Job drawing, mm, ordinate dimensions from the low corner. One solid piece. A direction names the side the tool comes from. Round coordinates to 2 decimals unless told otherwise and drop trailing zeros. Loops run counter-clockwise (first coordinate to the right, second up) from the corner with the lowest first, then second, coordinate; pieces in that order, holes last. Notation, with made-up numbers: M 13.25,77.25 L 33.25,77.25 A21 ccw 33.25,92.25 Z; hole C -24.75,77 d7. An arc over 180 degrees is marked long. Use a Markdown table: item, result. Add a question column.
(1) Flat gauge pins, fed straight in: P1, Ø1.8, axis at x = 20, z = 12.5, coming from the +Y side; P2, Ø7, axis at x = 20, z = 11, coming from the -Y side; P3, Ø4.5, axis at x = 7, y = 5.5, coming from the +Z side; P4, Ø2, axis at x = 22.5, y = 9, coming from the +Z side. Where does each tip first touch, or does it go through?
(2) Band-saw the part on C-C, the plane y = 3.5. Write the cut outline in (x, z).
(3) Which spindle directions (+Z, -Z, +X, -X, +Y, -Y) get a long thin tool onto all of the face, cutting with end or side? Do the marked faces 4, 5, 6 and 7. Say none if no direction does.
(4) Two-plate mould, pull along Z, no slides. Class the marked faces 1, 2 and 3: released by +Z, released by -Z, zero draft, split by the parting line, or undercut.
(5) Band-saw the part on B-B, the plane z = 11. Give the number of separate pieces and of enclosed holes in the cut face, and give its area (3 significant figures).
(6) Band-saw the part on A-A, the plane x = 5. Write the cut outline in (y, z).
(7) Wall check: L1, parallel to X at y = 9.3, z = 11; L2, parallel to X at y = 2, z = 11; L3, parallel to X at y = 4.75, z = 8.25. Give the ranges that are in metal, low to high.
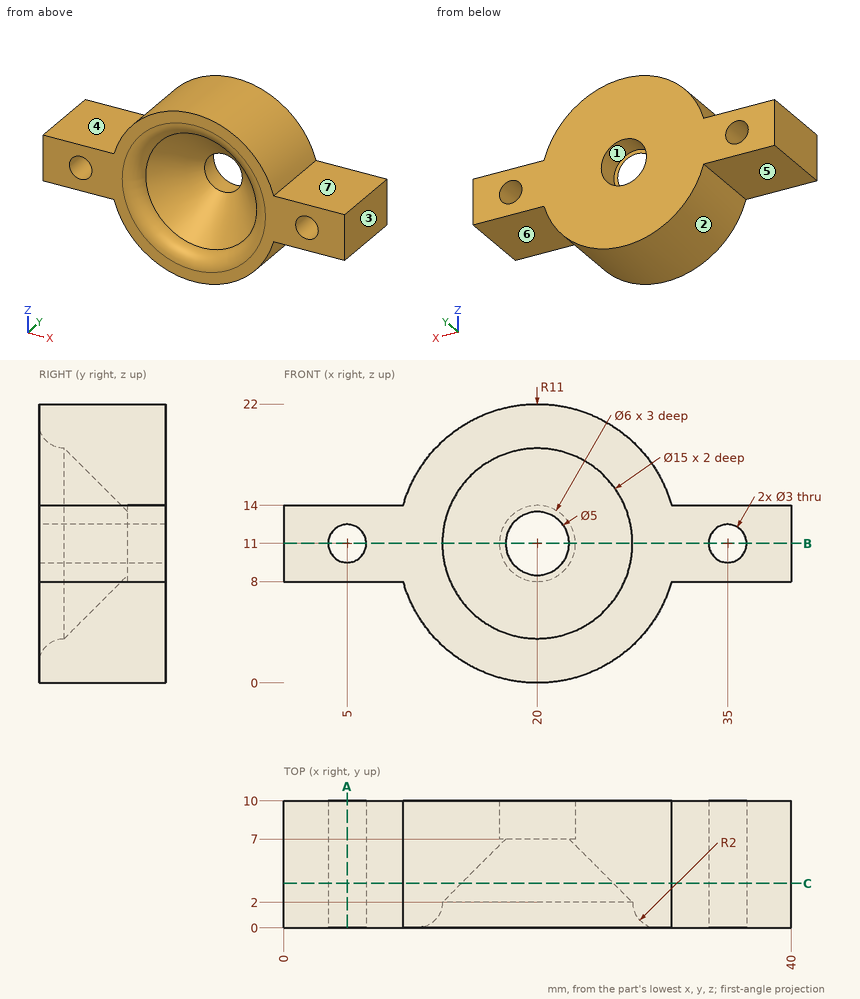
Return value:
| question | item | result |
|---|---|---|
| 1 | P1 | through |
| 1 | P2 | y = 6 |
| 1 | P3 | z = 14 |
| 1 | P4 | z = 21.9 |
| 2 | outline | M 0,8 L 9.42,8 A11 ccw 30.58,8 L 40,8 L 40,14 L 30.58,14 A11 ccw 9.42,14 L 0,14 Z; hole C 5,11 d3; hole C 20,11 d12; hole C 35,11 d3 |
| 3 | face 4 | +Z, -X, +Y, -Y |
| 3 | face 5 | -Z, -X, +Y, -Y |
| 3 | face 6 | -Z, +X, +Y, -Y |
| 3 | face 7 | +Z, +X, +Y, -Y |
| 4 | face 1 | undercut |
| 4 | face 2 | released by -Z |
| 4 | face 3 | zero draft |
| 5 | separate pieces | 4 |
| 5 | enclosed holes | 0 |
| 5 | area | 240 mm^2 |
| 6 | outline | M 0,8 L 10,8 L 10,9.5 L 0,9.5 Z; M 0,12.5 L 10,12.5 L 10,14 L 0,14 Z |
| 7 | L1 | 0 to 3.5, 6.5 to 17, 23 to 33.5, 36.5 to 40 |
| 7 | L2 | 0 to 3.5, 6.5 to 12.5, 27.5 to 33.5, 36.5 to 40 |
| 7 | L3 | 0 to 16.13, 23.87 to 40 |
